Geometry: final body of the model. Coordinates: model frame, mm. Round coordinates to 2 decimals unless told otherwise and drop trailing zeros. Order: outer loops, then holes, each group sorted by start corner. A loop starts at its lowest first (then second) coordinate and runs counter-clockwise, first axis right, second up. Notation, with made-up numbers: (-25.75, 22.25) -> (2.25, 22.25) arc R23 ccw to (2.25, 37.25) -> close; hole circle Ø4 at (34.5, -32.75). An arc over 180 degrees is marked (long way). Put each result on its own line as item: value.
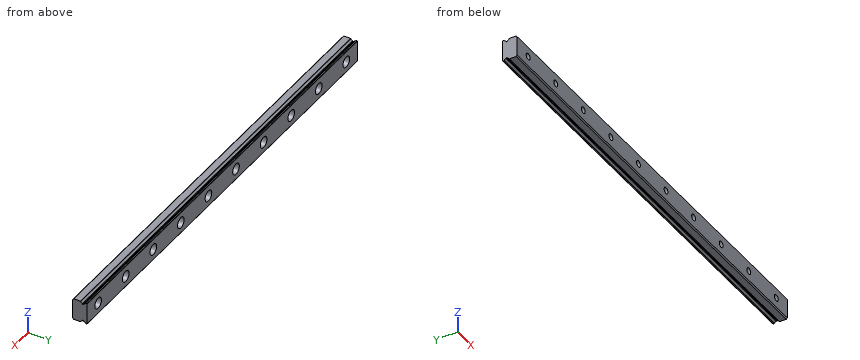
```python
from build123d import *

# Parameters (mm, degrees)
SKETCH_1_W                   = 245
SKETCH_1_H                   = 12
EXTRUDE_1_DEPTH              = 8
CUT_EXTRUDE_1_DEPTH          = 246.106099475
CUT_EXTRUDE_2_DEPTH          = 246.106099475
CUT_EXTRUDE_3_DEPTH          = 246.106099475
CUT_EXTRUDE_4_DEPTH          = 246.106099475
CUT_EXTRUDE_5_DEPTH          = 246.106099475
CUT_EXTRUDE_6_DEPTH          = 246.106099475
HOLE_WIZARD_M3_1_D           = 3.5
HOLE_WIZARD_M3_1_CBORE_D     = 5.9999
HOLE_WIZARD_M3_1_CBORE_DEPTH = 4.5
CHAMFER_1_SIZE               = 0.6
FILLET_1_R                   = 0.2


with BuildPart() as part:
    # 草图1 → 凸台-拉伸1 (new body)
    with BuildSketch(Plane(origin=(0, 4, 0), x_dir=(1, 0, 0), z_dir=(0, 1, 0))):
        Rectangle(SKETCH_1_W, SKETCH_1_H)
    extrude(amount=-EXTRUDE_1_DEPTH)

    # 草图2 → 切除-拉伸1 (cut, through all)
    with BuildSketch(Plane(origin=(122.5, 0, 0), x_dir=(0, 0, -1), z_dir=(1, 0, 0))):
        with BuildLine():
            Line((6, 1.51), (6, 2.01))
            Line((6, 2.01), (4.8, 2.01))
            ThreePointArc((4.8, 2.01), (4.55, 1.76), (4.8, 1.51))
            Line((4.8, 1.51), (6, 1.51))
        make_face()
    extrude(amount=-CUT_EXTRUDE_1_DEPTH, mode=Mode.SUBTRACT)

    # 草图3 → 切除-拉伸2 (cut, through all)
    with BuildSketch(Plane(origin=(122.5, 0, 0), x_dir=(0, 0, -1), z_dir=(1, 0, 0))):
        with BuildLine():
            Line((6, 2.01), (6, 3.111111))
            ThreePointArc((6, 3.111111), (5.367595703, 2.693428684), (5.04, 2.01))
            Line((5.04, 2.01), (6, 2.01))
        make_face()
    extrude(amount=-CUT_EXTRUDE_2_DEPTH, mode=Mode.SUBTRACT)

    # 草图4 → 切除-拉伸3 (cut, through all)
    with BuildSketch(Plane(origin=(122.5, 0, 0), x_dir=(0, 0, -1), z_dir=(1, 0, 0))):
        with BuildLine():
            Line((6, 1.51), (5.04, 1.51))
            ThreePointArc((5.04, 1.51), (5.367595703, 0.826571316), (6, 0.408889))
            Line((6, 0.408889), (6, 1.51))
        make_face()
    extrude(amount=-CUT_EXTRUDE_3_DEPTH, mode=Mode.SUBTRACT)

    # 草图5 → 切除-拉伸4 (cut, through all)
    with BuildSketch(Plane(origin=(122.5, 0, 0), x_dir=(0, 0, -1), z_dir=(1, 0, 0))):
        with BuildLine():
            Line((-6, 2.01), (-6, 1.51))
            Line((-6, 1.51), (-4.8, 1.51))
            ThreePointArc((-4.8, 1.51), (-4.55, 1.76), (-4.8, 2.01))
            Line((-4.8, 2.01), (-6, 2.01))
        make_face()
    extrude(amount=-CUT_EXTRUDE_4_DEPTH, mode=Mode.SUBTRACT)

    # 草图6 → 切除-拉伸5 (cut, through all)
    with BuildSketch(Plane(origin=(122.5, 0, 0), x_dir=(0, 0, -1), z_dir=(1, 0, 0))):
        with BuildLine():
            Line((-6, 1.51), (-6, 0.408889))
            ThreePointArc((-6, 0.408889), (-5.367595703, 0.826571316), (-5.04, 1.51))
            Line((-5.04, 1.51), (-6, 1.51))
        make_face()
    extrude(amount=-CUT_EXTRUDE_5_DEPTH, mode=Mode.SUBTRACT)

    # 草图7 → 切除-拉伸6 (cut, through all)
    with BuildSketch(Plane(origin=(122.5, 0, 0), x_dir=(0, 0, -1), z_dir=(1, 0, 0))):
        with BuildLine():
            Line((-6, 2.01), (-5.04, 2.01))
            ThreePointArc((-5.04, 2.01), (-5.367595703, 2.693428684), (-6, 3.111111))
            Line((-6, 3.111111), (-6, 2.01))
        make_face()
    extrude(amount=-CUT_EXTRUDE_6_DEPTH, mode=Mode.SUBTRACT)

    # M3 六角头机械螺钉的柱形沉头孔1 (through all)
    with Locations(Plane(origin=(0, 4, 0), x_dir=(1, 0, 0), z_dir=(0, 1, 0))):
        with Locations((-112.5, 0), (-87.5, 0), (-62.5, 0), (-37.5, 0), (-12.5, 0), (12.5, 0), (37.5, 0), (62.5, 0), (87.5, 0), (112.5, 0)):
            CounterBoreHole(HOLE_WIZARD_M3_1_D / 2, HOLE_WIZARD_M3_1_CBORE_D / 2, HOLE_WIZARD_M3_1_CBORE_DEPTH)

    # 倒角1
    chamfer_1_edges = [part.edges().sort_by_distance(p)[0] for p in [
        (0, -4, -6),
        (0, -4, 6),
    ]]
    chamfer(chamfer_1_edges, length=CHAMFER_1_SIZE)

    # 圆角1
    fillet_1_edges = [part.edges().sort_by_distance(p)[0] for p in [
        (0, 2.01, -5.04),
        (0, 3.111111, -6),
        (0, 0.408889, -6),
        (0, 1.51, -5.04),
        (0, 4, -6),
        (0, 4, 6),
        (0, 1.51, 5.04),
        (0, 0.408889, 6),
        (0, 3.111111, 6),
        (0, 2.01, 5.04),
    ]]
    fillet(fillet_1_edges, radius=FILLET_1_R)


solid = part.part
```
1. Contact query for flat-ended pins moving along their axis: P1, Ø3, axis at x = -88.5, z = 0.5, coming from the +Y side; P2, Ø3, axis at x = -7, y = 2.5, coming from the +Z side. Output: stop coordinate, or through.
Ans:
P1: y = -0.5
P2: z = 6
2. Cut plane A-A on x = -1. Return loops of the section in (y, z), and give its area (3 significant figures).
Ans:
outline: (-4, -5.4) -> (-3.4, -6) -> (0.27, -6) arc R0.2 ccw to (0.45, -5.88) arc R1.42 cw to (1.37, -5.07) arc R0.2 ccw to (1.51, -4.88) -> (1.51, -4.8) arc R0.25 cw to (2.01, -4.8) -> (2.01, -4.88) arc R0.2 ccw to (2.15, -5.07) arc R1.42 cw to (3.07, -5.88) arc R0.2 ccw to (3.25, -6) -> (3.8, -6) arc R0.2 ccw to (4, -5.8) -> (4, 5.8) arc R0.2 ccw to (3.8, 6) -> (3.25, 6) arc R0.2 ccw to (3.07, 5.88) arc R1.42 cw to (2.15, 5.07) arc R0.2 ccw to (2.01, 4.88) -> (2.01, 4.8) arc R0.25 cw to (1.51, 4.8) -> (1.51, 4.88) arc R0.2 ccw to (1.37, 5.07) arc R1.42 cw to (0.45, 5.88) arc R0.2 ccw to (0.27, 6) -> (-3.4, 6) -> (-4, 5.4) -> close
area: 91.3 mm²
3. Material intervals for probe 1 along Y at (x, z) = (3.5, -4.75); probe 2 along Z at (x, y) = (87.5, -3.15); probe 3 along Z at (x, y) = (87.5, 0.85), sorted ascending.
Ans:
probe 1: -4 to 1.52, 2 to 4
probe 2: -6 to -1.75, 1.75 to 6
probe 3: -5.35 to -3, 3 to 5.35
